```python
from build123d import *

# Parameters (mm, degrees)
SKETCH_1_W          = 35.68
SKETCH_1_H          = 20
SKETCH_1_R          = 1.5
EXTRUDE_1_DEPTH     = 5
EXTRUDE_2_DEPTH     = 10
SKETCH_1_5_R        = 1.5
CUT_EXTRUDE_1_DEPTH = 1.5
EXTRUDE_4_DEPTH     = 25
CUT_EXTRUDE_3_REACH = 46.7
SKETCH_3_R          = 2.5
EXTRUDE_START       = -10
EXTRUDE_3_DEPTH     = 20
CHAMFER_1_SIZE      = 3.1
CHAMFER_2_SIZE      = 5


with BuildPart() as part:
    # 草图1 → 凸台-拉伸1 (new body)
    with BuildSketch(Plane(origin=(0, 0, 0), x_dir=(1, 0, 0), z_dir=(0, 1, 0))):
        with Locations((17.84, 0)):
            Rectangle(SKETCH_1_W, SKETCH_1_H)
        with Locations(Location((25.68, 0, 0), (0, 0, 270))):
            Circle(SKETCH_1_R, mode=Mode.SUBTRACT)
    extrude(amount=EXTRUDE_1_DEPTH)

    # 草图1<4> → 凸台-拉伸2 (add)
    with BuildSketch(Plane(origin=(0, 0, 0), x_dir=(1, 0, 0), z_dir=(0, 1, 0))):
        Polygon((25.68, 5), (35.68, 5), (35.68, 10), (5, 10), (5, 5), align=None)
        Polygon((35.68, -10), (35.68, -5), (25.68, -5), (5, -5), (5, -10), align=None)
    extrude(amount=EXTRUDE_2_DEPTH)

    # 草图1<5> → 切除-拉伸1 (cut)
    with BuildSketch(Plane(origin=(0, 0, 0), x_dir=(1, 0, 0), z_dir=(0, 1, 0))):
        Polygon((24.09228676, -2.75), (27.26771324, -2.75), (28.855426481, 0), (27.26771324, 2.75), (24.09228676, 2.75), (22.504573519, 0), align=None)
        with Locations(Location((25.68, 0, 0), (0, 0, 270))):
            Circle(SKETCH_1_5_R, mode=Mode.SUBTRACT)
    extrude(amount=CUT_EXTRUDE_1_DEPTH, mode=Mode.SUBTRACT)

    # 草图1<6> → 凸台-拉伸4 (add)
    with BuildSketch(Plane(origin=(0, 0, 0), x_dir=(1, 0, 0), z_dir=(0, 1, 0))):
        Polygon((5, -5), (5, 5), (5, 10), (0, 10), (0, -10), (5, -10), align=None)
    extrude(amount=EXTRUDE_4_DEPTH)

    # 草图3 → 切除-拉伸3 (cut, up to next)
    with BuildSketch(Plane(origin=(0, 0, 0), x_dir=(0, 0, -1), z_dir=(1, 0, 0)), mode=Mode.PRIVATE) as cut_extrude_3_sk1:
        with Locations((0, 20)):
            Circle(SKETCH_3_R)
    cut_extrude_3_tool1 = extrude(cut_extrude_3_sk1.sketch, amount=CUT_EXTRUDE_3_REACH, mode=Mode.PRIVATE) & part.part
    add(cut_extrude_3_tool1.solids().sort_by_distance((0, 20, 0))[0], mode=Mode.SUBTRACT)

    # 草图2 → 凸台-拉伸3 (add)
    with BuildSketch(Plane.XY.offset(EXTRUDE_START)):
        Polygon((0, 3.1), (-2, 3.1), (-2, 5.4), (-3.6, 5.4), (-6, 3), (-6, -3), (-3.6, -5.4), (-2, -5.4), (-2, -3.1), (0, -3.1), align=None)
    extrude(amount=EXTRUDE_3_DEPTH)

    # 倒角1
    chamfer_1_edges = [part.edges().sort_by_distance(p)[0] for p in [
        (0, 0, 0),
    ]]
    chamfer(chamfer_1_edges, length=CHAMFER_1_SIZE - 0.0001)  # a hair under: the kernel refuses the full size

    # 倒角2
    chamfer_2_edges = [part.edges().sort_by_distance(p)[0] for p in [
        (5, 5, 0),
    ]]
    chamfer(chamfer_2_edges, length=CHAMFER_2_SIZE)


solid = part.part
```
Here's how the part is built. I have some questions about the finished solid (model axes, mm). A direction names the side the tool comes from. Coordinates: 2 decimals unless noted, no trailing zeros. Loops run counter-clockwise (first coordinate to the right, second up) from the corner with the lowest first, then second, coordinate; pieces in that order, holes last. Notation, with made-up numbers: (89.25, 83) - (125.25, 83) arc R24 ccw to (125.25, 106) - close; hole circle Ø1 at (44.25, -17). An arc over 180 degrees is marked (long way). Answer as CSV lines item,"result".
Q1. If I drill on L1, parallel to X at y = 4, z = 0; L2, parallel to X at y = 3.6, z = 0; L3, parallel to Z at x = 1.4, y = 20, over which ranges is the centre line in solid material (lowest first)? Write a range as [from, to].
Response:
L1,"[-5, -2], [0, 24.18], [27.18, 35.68]"
L2,"[-5.4, -2], [0, 24.18], [27.18, 35.68]"
L3,"[-10, -2.5], [2.5, 10]"
Q2. We'd pull the mould along X, two halves only. Please class faces 1 (the face through (-5, 4, 0)), 2 (the face through (-3, 5.4, 0)), 3 (the face through (26, 1, -2.75)): pulls with the +X half, pulls with the -X half, needs draft (parallel to the pull), parting line crosses it, or undercut.
Response:
face 1,"pulls with the -X half"
face 2,"needs draft"
face 3,"undercut"
Q3. If we section it at A-A, the plane y = 4: Write out the boundary of the cut face in (x, z).
Response:
outline,"(-5, -10) - (-2, -10) - (-2, 10) - (-5, 10) - close; (0, -10) - (35.68, -10) - (35.68, 10) - (0, 10) - close; hole circle Ø3 at (25.68, 0)"
Q4. For faces 4 (the face through (23.31, 0.74, -1.394)), 5 (the face through (19, 0, 0)), 6 (the face through (23, 5, 0)), which set-ups out of +Z, -Z, +X, -X, +Y, -Y let a thin tool reach every point of the face, with its end or its side?
Response:
face 4,"-Y"
face 5,"+Z, -Z, +X, -Y"
face 6,"+X, +Y"
Q5. If we section it at D-D, the plane x = 8: Write out the boundary of the cut face in (y, z).
Response:
outline,"(0, -10) - (10, -10) - (10, -5) - (7, -5) - (7, 5) - (10, 5) - (10, 10) - (0, 10) - close"
Q6. For pin 1 (2.5 mm diameter, centred on x = 25.5, z = 7.5, fed in from +Y); pin 2 (8 mm diameter, centred on y = 6.5, z = 2.5, fed in from +X); pin 3 (2 mm diameter, centred on y = 14.5, z = 4, fed in from +X); pin 4 (4 mm diameter, centred on x = 8, z = 4.5, fed in from -Y), each with a flat end and sliding along its axis, tell me the tip position at first contact or that it passes through.
Response:
pin 1,"y = 10"
pin 2,"x = 35.68"
pin 3,"x = 5"
pin 4,"y = 0"
Q7. If we section it at B-B, the plane x = 25.68: Write out the boundary of the cut face in (y, z), and give its area (3 significant figures).
Response:
outline,"(0, -10) - (10, -10) - (10, -5) - (5, -5) - (5, -1.5) - (1.5, -1.5) - (1.5, -2.75) - (0, -2.75) - close; (0, 2.75) - (1.5, 2.75) - (1.5, 1.5) - (5, 1.5) - (5, 5) - (10, 5) - (10, 10) - (0, 10) - close"
area,"131 mm2"
